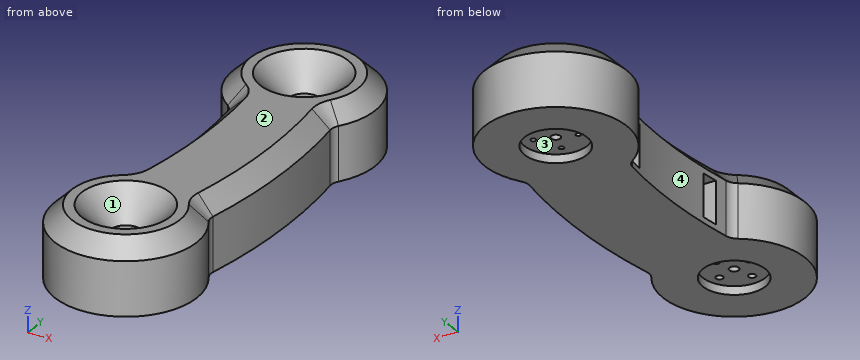
```python
from build123d import *

# Parameters (mm, degrees)
BOSS_EXTRUDE2_DEPTH = 12.5
SKETCH2_R           = 1.65
CUT_EXTRUDE1_DEPTH  = 183.452259897
SKETCH4_R           = 11
CUT_EXTRUDE3_DEPTH  = 3
CHAMFER1_SIZE       = 6
SKETCH32_R          = 1.275
CUT_EXTRUDE6_DEPTH  = 8
SKETCH34_R          = 0.9
CUT_EXTRUDE7_DEPTH  = 8
SKETCH44_R          = 5.5
CUT_EXTRUDE8_DEPTH  = 19
CHAMFER2_SIZE       = 10
CUT_SWEEP1_START    = -10.5
CUT_SWEEP1_DEPTH    = 15


# Read off the part's stored shape, not the designer's step: Cut-Sweep1
with BuildPart() as part:
    # Sketch1 → Boss-Extrude2 (new, symmetric)
    with BuildSketch(Plane.XY):
        with BuildLine():
            ThreePointArc((20.986978603, -67.578728182), (-4.772573404, -29.453707497), (-14.365917101, -74.454146144))
            ThreePointArc((-14.365917101, -74.454146144), (-12.975360601, -75.93457639), (-12.28837595, -77.845956305))
            ThreePointArc((-12.28837595, -77.845956305), (-10.448341727, -103.99393046), (-12.28837595, -130.141904615))
            ThreePointArc((-12.28837595, -130.141904615), (-12.975360601, -132.05328453), (-14.365917101, -133.533714776))
            ThreePointArc((-14.365917101, -133.533714776), (-4.772573404, -178.534153424), (20.986978603, -140.409132739))
            ThreePointArc((20.986978603, -140.409132739), (20.288835581, -138.708883787), (20.252226745, -136.871246725))
            ThreePointArc((20.252226745, -136.871246725), (22.969651044, -103.99393046), (20.252226745, -71.116614196))
            ThreePointArc((20.252226745, -71.116614196), (20.288835581, -69.278977134), (20.986978603, -67.578728182))
        make_face()
    extrude(amount=BOSS_EXTRUDE2_DEPTH, both=True)

    # Sketch2 → Cut-Extrude1 (cut, through all)
    with BuildSketch(Plane.XY.offset(12.5)):
        with Locations((0, -53.99393046)):
            Circle(SKETCH2_R)
        with Locations((0, -153.99393046)):
            Circle(SKETCH2_R)
    extrude(amount=-CUT_EXTRUDE1_DEPTH, mode=Mode.SUBTRACT)

    # Sketch4 → Cut-Extrude3 (cut)
    with BuildSketch(Plane(origin=(0, 0, -12.5), x_dir=(-1, 0, 0), z_dir=(0, 0, -1))):
        with Locations((0, -53.99393046)):
            Circle(SKETCH4_R)
        with Locations((0, -153.99393046)):
            Circle(SKETCH4_R)
    extrude(amount=-CUT_EXTRUDE3_DEPTH, mode=Mode.SUBTRACT)

    # Chamfer1
    chamfer1_edges = [part.edges().sort_by_distance(p)[0] for p in [
        (20.288835581, -69.278977134, 12.5),
        (-4.772573404, -29.453707497, 12.5),
        (-12.975360601, -75.93457639, 12.5),
        (-10.448341727, -103.99393046, 12.5),
        (-12.975360601, -132.05328453, 12.5),
        (-4.772573404, -178.534153424, 12.5),
        (20.288835581, -138.708883787, 12.5),
        (22.969651044, -103.99393046, 12.5),
    ]]
    chamfer(chamfer1_edges, length=CHAMFER1_SIZE)

    # Sketch32 → Cut-Extrude6 (cut)
    with BuildSketch(Plane(origin=(0, 0, -12.5), x_dir=(-1, 0, 0), z_dir=(0, 0, -1))):
        with Locations((-2.194575755, -147.346838069)):
            Circle(SKETCH32_R)
        with Locations((6.647092391, -151.799354705)):
            Circle(SKETCH32_R)
        with Locations((-6.647092391, -156.188506215)):
            Circle(SKETCH32_R)
        with Locations((2.194575755, -160.641022851)):
            Circle(SKETCH32_R)
    extrude(amount=-CUT_EXTRUDE6_DEPTH, mode=Mode.SUBTRACT)

    # Sketch34 → Cut-Extrude7 (cut)
    with BuildSketch(Plane(origin=(0, 0, -9.5), x_dir=(-1, 0, 0), z_dir=(0, 0, -1))):
        with Locations((-6.647092391, -51.799354705)):
            Circle(SKETCH34_R)
        with Locations((2.194575755, -47.346838069)):
            Circle(SKETCH34_R)
        with Locations((6.647092391, -56.188506215)):
            Circle(SKETCH34_R)
        with Locations((-2.194575755, -60.641022851)):
            Circle(SKETCH34_R)
        with Locations((-2.194575755, -147.346838069)):
            Circle(SKETCH34_R)
        with Locations((-6.647092391, -156.188506215)):
            Circle(SKETCH34_R)
        with Locations((2.194575755, -160.641022851)):
            Circle(SKETCH34_R)
        with Locations((6.647092391, -151.799354705)):
            Circle(SKETCH34_R)
    extrude(amount=-CUT_EXTRUDE7_DEPTH, mode=Mode.SUBTRACT)

    # Sketch44 → Cut-Extrude8 (cut)
    with BuildSketch(Plane.XY.offset(12.5)):
        with Locations((0, -53.99393046)):
            Circle(SKETCH44_R)
        with Locations((0, -153.99393046)):
            Circle(SKETCH44_R)
    extrude(amount=-CUT_EXTRUDE8_DEPTH, mode=Mode.SUBTRACT)

    # Chamfer2
    chamfer2_edges = [part.edges().sort_by_distance(p)[0] for p in [
        (-5.5, -53.99393046, 12.5),
        (-5.5, -153.99393046, 12.5),
    ]]
    chamfer(chamfer2_edges, length=CHAMFER2_SIZE)

    # Cut-Sweep1 outline → Cut-Sweep1 (cut)
    with BuildSketch(Plane.XY.offset(CUT_SWEEP1_START)):
        with BuildLine():
            Line((-2.026503985, -76.769481595), (-12.443832541, -76.769481595))
            ThreePointArc((-12.443832541, -76.769481595), (-12.365320392, -77.307605752), (-12.28837595, -77.845956305))
            ThreePointArc((-12.28837595, -77.845956305), (-11.957138623, -80.305626129), (-11.658625557, -82.769481595))
            Line((-11.658625557, -82.769481595), (-2.026503985, -82.769481595))
            ThreePointArc((-2.026503985, -82.769481595), (1.509029921, -84.233947689), (2.973496015, -87.769481595))
            Line((2.973496015, -87.769481595), (2.973496015, -114.4079942))
            ThreePointArc((2.973496015, -114.4079942), (1.509029921, -117.943528106), (-2.026503985, -119.4079942))
            Line((-2.026503985, -119.4079942), (-11.085695711, -119.4079942))
            ThreePointArc((-11.085695711, -119.4079942), (-11.358836079, -122.410395034), (-11.680419149, -125.4079942))
            Line((-11.680419149, -125.4079942), (-2.026503985, -125.4079942))
            ThreePointArc((-2.026503985, -125.4079942), (5.751670608, -122.186168793), (8.973496015, -114.4079942))
            Line((8.973496015, -114.4079942), (8.973496015, -87.769481595))
            ThreePointArc((8.973496015, -87.769481595), (5.751670608, -79.991307002), (-2.026503985, -76.769481595))
        make_face()
    extrude(amount=CUT_SWEEP1_DEPTH, mode=Mode.SUBTRACT)


solid = part.part
```
Work out the finished part from the listing and answer in its coordinate system (mm). Face numbers are marked on the shaded views. A direction names the side the tool comes from. Give positions to 0.01 mm unless a question says otherwise; leave off trailing zeros. Loops run counter-clockwise (first coordinate to the right, second up) from the corner with the lowest first, then second, coordinate; pieces in that order, holes last. Notation, with made-up numbers: (34, 62) - (86, 62) arc R35 cw to (86, 99) - close; hole circle Ø10 at (42.25, 77). An arc over 180 degrees is marked (long way). One line per question, with ' | ' between items.
(1) The part is cut by section A-A (z = 0.75). Write down the section's boundary in (x, y), then the cut area to 3 significant figures.
Recorded:
outline: (-14.37, -133.53) arc R25 ccw (long way) to (20.99, -140.41) arc R5 cw to (20.25, -136.87) arc R200.25 ccw to (20.25, -71.12) arc R5 cw to (20.99, -67.58) arc R25 ccw (long way) to (-14.37, -74.45) arc R5 cw to (-12.29, -77.85) arc R186.71 ccw to (-12.44, -76.77) - (-2.03, -76.77) arc R11 cw to (8.97, -87.77) - (8.97, -114.41) arc R11 cw to (-2.03, -125.41) - (-11.68, -125.41) arc R186.71 cw to (-12.29, -130.14) arc R5 cw to start; (-11.66, -82.77) arc R186.71 cw to (-11.09, -119.41) - (-2.03, -119.41) arc R5 ccw to (2.97, -114.41) - (2.97, -87.77) arc R5 ccw to (-2.03, -82.77) - close; hole circle Ø11 at (0, -153.99); hole circle Ø11 at (0, -53.99) | area: 5,150 mm²
(2) A tool of negligible diameter and unlimited length cuts with its end or side. For the marked faces 3 and 4, from which of +Z, -Z, +X, -X, +Y, -Y can it reach the whole face along a straight path? Write none if from no direction.
Recorded:
face 3: -Z | face 4: +Z, -Z, -X
(3) The mould has two halves that part along Y. Classify the marked faces 1 and 2: +Y half, -Y half, draft (parallel to the pull), parting line (faces both ways), or undercut.
Recorded:
face 1: undercut | face 2: draft
(4) Straight lines are drawn through the part: probe 1 along Y at (x, z) = (0, -11.6); probe 2 along Z at (x, y) = (7.5, -110); probe 3 along Y at (x, z) = (0, -4). For each, find the intervals that lie inside material, in ascending order.
Recorded:
probe 1: y = -178.99 to -164.99, -142.99 to -64.99, -42.99 to -28.99 | probe 2: z = -12.5 to -10.5, 4.5 to 12.5 | probe 3: y = -178.99 to -159.49, -148.49 to -125.22, -118.98 to -83.2, -76.96 to -59.49, -48.49 to -28.99
(5) Each of these flat-tipped pins is pushed along its axis until it touches: pin 1 Ø3 at (y, z) = (-76.5, 3.5) entering from -X; pin 2 Ø4 at (x, z) = (-6.5, 0.5) entering from +Y; pin 3 Ø3 at (x, z) = (-14.5, -10) entering from -Y. Where does it stop, or does it pass through?
Recorded:
pin 1: stops at x = -13.71 | pin 2: stops at y = -29.4 | pin 3: stops at y = -175.35
